The listing builds one solid part. Answer for the finished solid, in the listing's coordinates (mm). Face numbers are marked on the shaded views. Give positions to 0.01 mm unless a question says otherwise; leave off trailing zeros. Loops run counter-clockwise (first coordinate to the right, second up) from the corner with the lowest first, then second, coordinate; pieces in that order, holes last.
Item 1: Section A-A, the plane x = 0 is taken. Give the vertices of the cut face in (y, z), and give its area (3 significant figures).
Item 2: The mould has two halves that part along X. Classify the marked faces 1, 2, 3 and 4: pulls with the +X half, pulls with the -X half, needs draft (parallel to the pull), parting line crosses it, or undercut.
Item 3: Section C-C, the plane x = -11.5 is taken. Give the number of separate pieces and of enclosed holes in the cut face, and give its area (3 significant figures).
Item 4: Each of these flat-tipped pins is pushed along its axis until it touches: pin 1 Ø10 at (x, z) = (9.5, 12) entering from +Y; pin 2 Ø1 at (y, z) = (-46, 3.5) entering from +X; pin 3 Ø8 at (x, z) = (-11.5, 4) entering from -Y. Where does it stop, or does it pass through?
Item 5: Section B-B, the plane z = 11 is taken. Give the vertices of the cut face in (x, y), and give its area (3 significant figures).
Item 6: Section D-D, the plane x = 23 is taken. Give the vertices of the cut face in (y, z), and give its area (3 significant figures).
Item 7: Consider line 1 along Y through (x, z) = (-16.5, 8.5); line 2 along Y through (x, z) = (-9.5, 5); line 3 along X through (y, z) = (-39, 11). Determine where each line is inside the solid, lowest interval first.
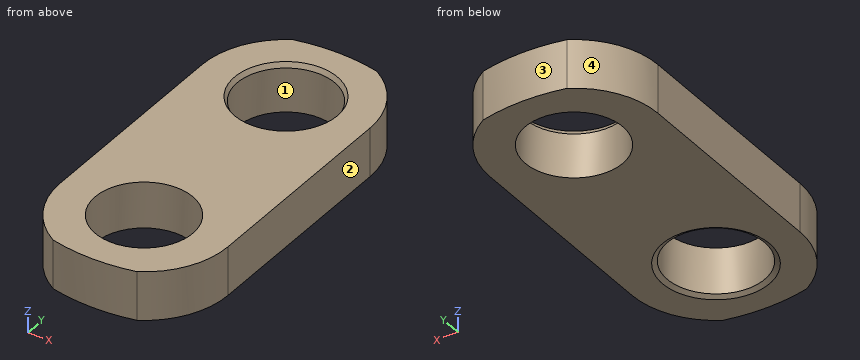
from build123d import *

# Parameters (mm, degrees)
SKETCH_1_R      = 18
EXTRUDE_1_DEPTH = 18
CHAMFER_1_SIZE  = 1
CHAMFER_1_SIZE2 = 1.732050808
CHAMFER_2_SIZE  = 1
CHAMFER_2_SIZE2 = 1.732050808


with BuildPart() as part:
    # Эскиз1 → Бобышка-Вытянуть1 (new body)
    with BuildSketch(Plane.XY):
        with BuildLine():
            Line((-31, 39), (-31, -39))
            ThreePointArc((-31, -39), (-26.846787517, -54.5), (-15.5, -65.846787517))
            ThreePointArc((-15.5, -65.846787517), (0, -67.64650343), (15.5, -65.846787517))
            ThreePointArc((15.5, -65.846787517), (26.846787517, -54.5), (31, -39))
            Line((31, -39), (31, 39))
            ThreePointArc((31, 39), (26.846787517, 54.5), (15.5, 65.846787517))
            ThreePointArc((15.5, 65.846787517), (0, 67.64650343), (-15.5, 65.846787517))
            ThreePointArc((-15.5, 65.846787517), (-26.846787517, 54.5), (-31, 39))
        make_face()
        with Locations((0, 39)):
            Circle(SKETCH_1_R, mode=Mode.SUBTRACT)
        with Locations(Location((0, -39, 0), (0, 0, 180))):
            Circle(SKETCH_1_R, mode=Mode.SUBTRACT)
    extrude(amount=EXTRUDE_1_DEPTH)

    # Фаска1
    chamfer_1_edges = [part.edges().sort_by_distance(p)[0] for p in [
        (-18, 39, 18),
    ]]
    chamfer_1_side = [part.faces().sort_by_distance(p)[0] for p in [
        (0, 0, 18),
    ]]
    chamfer(chamfer_1_edges, length=CHAMFER_1_SIZE, length2=CHAMFER_1_SIZE2, reference=chamfer_1_side[0])

    # Фаска2
    chamfer_2_edges = [part.edges().sort_by_distance(p)[0] for p in [
        (18, -39, 0),
    ]]
    chamfer_2_side = [part.faces().sort_by_distance(p)[0] for p in [
        (18, -39, 9),
    ]]
    chamfer(chamfer_2_edges, length=CHAMFER_2_SIZE, length2=CHAMFER_2_SIZE2, reference=chamfer_2_side[0])


solid = part.part
Worked answers:
1. outline: (-67.65, 0) - (-58.73, 0) - (-57, 1) - (-57, 18) - (-67.65, 18) - close; (-21, 1) - (-19.27, 0) - (21, 0) - (21, 16.27) - (20, 18) - (-21, 18) - close; (57, 0) - (67.65, 0) - (67.65, 18) - (58, 18) - (57, 16.27) - close
1. area: 1,140 mm2
2. face 1: undercut
2. face 2: pulls with the +X half
2. face 3: parting line crosses it
2. face 4: pulls with the -X half
3. separate pieces: 3
3. enclosed holes: 0
3. area: 1,400 mm2
4. pin 1: stops at y = 67.5
4. pin 2: stops at x = 30.31
4. pin 3: stops at y = -67.23
5. outline: (-31, -39) arc R31 ccw to (-15.5, -65.85) arc R67.65 ccw to (15.5, -65.85) arc R31 ccw to (31, -39) - (31, 39) arc R31 ccw to (15.5, 65.85) arc R67.65 ccw to (-15.5, 65.85) arc R31 ccw to (-31, 39) - close; hole circle Ø36 at (0, -39); hole circle Ø36 at (0, 39)
5. area: 5,720 mm2
6. outline: (-59.78, 0) - (59.78, 0) - (59.78, 18) - (-59.78, 18) - close
6. area: 2,150 mm2
7. line 1: y = -65.24 to -46.19, -31.81 to 31.81, 46.19 to 65.24
7. line 2: y = -66.98 to -54.29, -23.71 to 23.71, 54.29 to 66.98
7. line 3: x = -31 to -18, 18 to 31
